```python
from build123d import *

# Parameters (mm, degrees)
BOSS_EXTRUDE1_DEPTH = 3.5814
BOSS_EXTRUDE2_DEPTH = 3.5814
SKETCH4_R           = 7.95
CUT_EXTRUDE2_DEPTH  = 4.5814
CUT_EXTRUDE4_REACH  = 5.581
CUT_EXTRUDE5_REACH  = 5.581


with BuildPart() as part:
    # Sketch1 → Boss-Extrude1 (new body)
    with BuildSketch(Plane(origin=(0, 0, 0), x_dir=(1, 0, 0), z_dir=(0, 1, 0))):
        Polygon((-25.0063, -13.0482), (25.0063, -13.0482), (25.0063, -2.05), (1.7907, -2.05), (1.7907, 2.05), (9.398, 2.05), (1.7907, 7.13), (-1.7907, 7.13), (-9.398, 2.05), (-1.7907, 2.05), (-1.7907, -2.05), (-25.0063, -2.05), align=None)
    extrude(amount=BOSS_EXTRUDE1_DEPTH)

    # Sketch3 → Boss-Extrude2 (add)
    with BuildSketch(Plane(origin=(0, 3.5814, 0), x_dir=(1, 0, 0), z_dir=(0, 1, 0))):
        Polygon((-25.0063, -2.05), (-25.0063, -13.0482), (25.0063, -13.0482), (25.0063, -2.05), (1.7907, -2.05), (1.7907, 2.05), (9.398, 2.05), (1.7907, 7.13), (-1.7907, 7.13), (-9.398, 2.05), (-1.7907, 2.05), (-1.7907, -2.05), align=None)
        with BuildLine():
            Line((25.0063, -13.0482), (-25.0063, -13.0482))
            ThreePointArc((-25.0063, -13.0482), (-16.136037163, -25.01193231), (-2.111127058, -20.000510342))
            ThreePointArc((-2.111127058, -20.000510342), (0, -18.87286389), (2.111127058, -20.000510342))
            ThreePointArc((2.111127058, -20.000510342), (16.136037163, -25.01193231), (25.0063, -13.0482))
        make_face()
    extrude(amount=-BOSS_EXTRUDE2_DEPTH)

    # Sketch4 → Cut-Extrude2 (cut, through all)
    with BuildSketch(Plane(origin=(0, 3.5814, 0), x_dir=(1, 0, 0), z_dir=(0, 1, 0))):
        with Locations((-13.5, -13.0482)):
            Circle(SKETCH4_R)
        with Locations((13.5, -13.0482)):
            Circle(SKETCH4_R)
    extrude(amount=-CUT_EXTRUDE2_DEPTH, mode=Mode.SUBTRACT)

    # Sketch5 → Cut-Extrude4 (cut, up to next)
    with BuildSketch(Plane(origin=(0, 3.5814, 0), x_dir=(1, 0, 0), z_dir=(0, 1, 0)), mode=Mode.PRIVATE) as cut_extrude4_sk1:
        with BuildLine():
            Line((-3.25, -3.8), (3.25, -3.8))
            ThreePointArc((3.25, -3.8), (4.487436867, -4.312563133), (5, -5.55))
            Line((5, -5.55), (10.858126279, -5.55))
            ThreePointArc((10.858126279, -5.55), (7.011340813, -8.454747926), (5.55, -13.0482))
            Line((5.55, -13.0482), (-5.55, -13.0482))
            ThreePointArc((-5.55, -13.0482), (-7.011340813, -8.454747926), (-10.858126279, -5.55))
            Line((-10.858126279, -5.55), (-5, -5.55))
            ThreePointArc((-5, -5.55), (-4.487436867, -4.312563133), (-3.25, -3.8))
        make_face()
    cut_extrude4_tool1 = extrude(cut_extrude4_sk1.sketch, amount=-CUT_EXTRUDE4_REACH, mode=Mode.PRIVATE) & part.part
    add(cut_extrude4_tool1.solids().sort_by_distance((0, 3.5814, 8.325803))[0], mode=Mode.SUBTRACT)

    # Sketch6 → Cut-Extrude5 (cut, up to next)
    with BuildSketch(Plane(origin=(0, 3.5814, 0), x_dir=(1, 0, 0), z_dir=(0, 1, 0)), mode=Mode.PRIVATE) as cut_extrude5_sk1:
        with BuildLine():
            Line((-18.450280122, -2.05), (-25.0063, -2.05))
            Line((-25.0063, -2.05), (-25.0063, -13.0482))
            ThreePointArc((-25.0063, -13.0482), (-23.242950275, -6.64621203), (-18.450280122, -2.05))
        make_face()
    cut_extrude5_tool1 = extrude(cut_extrude5_sk1.sketch, amount=-CUT_EXTRUDE5_REACH, mode=Mode.PRIVATE) & part.part
    add(cut_extrude5_tool1.solids().sort_by_distance((-23.17616, 3.5814, 4.635288))[0], mode=Mode.SUBTRACT)
    # Sketch6 → Cut-Extrude5 (cut, up to next)
    with BuildSketch(Plane(origin=(0, 3.5814, 0), x_dir=(1, 0, 0), z_dir=(0, 1, 0)), mode=Mode.PRIVATE) as cut_extrude5_sk2:
        with BuildLine():
            Line((25.0063, -13.0482), (25.0063, -2.05))
            Line((25.0063, -2.05), (18.450280122, -2.05))
            ThreePointArc((18.450280122, -2.05), (23.242950275, -6.64621203), (25.0063, -13.0482))
        make_face()
    cut_extrude5_tool2 = extrude(cut_extrude5_sk2.sketch, amount=-CUT_EXTRUDE5_REACH, mode=Mode.PRIVATE) & part.part
    add(cut_extrude5_tool2.solids().sort_by_distance((23.17616, 3.5814, 4.635288))[0], mode=Mode.SUBTRACT)


solid = part.part
```
Check sheet for the modelled part. Datum: model origin and axes. Units: mm. A direction names the side the tool comes from. Round coordinates to 2 decimals unless told otherwise and drop trailing zeros. Write each loop counter-clockwise with the first axis right and the second up, starting at its lowest first coordinate (ties: lowest second). Pieces come first, ordered by that corner, then holes. Notation, with made-up numbers: M 17,-24.5 L 71,-24.5 A23 ccw 71,-0.5 Z; hole C 70.5,-33 d5. An arc over 180 degrees is marked long. Write item = value, one per line. Start each with the question number.
1. Release check for a two-part mould opening along X. For faces 6 (the flat face through (-2, 3.581, 14)), 7 (the flat face through (5.648, 1.766, -4.554)), 8 (the cylindrical face through (19.8, 1.8, 17.9)) record: pulls with the +X half, pulls with the -X half, needs draft (parallel to the pull), parting line crosses it, or undercut.
2. Tool access check on faces 1 (the flat face through (6, 2, -2.05)), 2 (the flat face through (-2, 0, 14)), 3 (the flat face through (0, 2, -7.13)), 4 (the flat face through (8, 2, 5.55)), 5 (the flat face through (-6, 2, -2.05)). Record the directions out of +Z, -Z, +X, -X, +Y, -Y that give a thin tool (end or side, any length) a straight path to the whole face; none if there is none.
3. Section check D-D, the plane z = 16. Record the cut outline in (x, y).
4. Section check A-A, the plane y = 1.3. Record the cut outline in (x, z), then the cut area to 3 significant figures.
5. Gauge pin test, flat ends, axial feed: pin 1 (2 mm diameter, centred on x = 13, y = 2.5, fed in from -Z); pin 2 (9.5 mm diameter, centred on x = -13.5, z = 13.05, fed in from +Y); pin 3 (1.8 mm diameter, centred on x = 0, y = 1, fed in from +Z); pin 4 (1.1 mm diameter, centred on x = -4.5, y = 1, fed in from +Z). Record the tip position at first contact, or that the pin passes through.
6. Scan lines: line 1 (X direction, y = 0.7, z = 13); line 2 (Z direction, x = -7.5, y = 3.05); line 3 (X direction, y = 1.05, z = 19.5). Record each from-to range of solid material in increasing order. Write a range as [from, to].
7. Section check B-B, the plane x = 17.5. Record the cut outline in (y, z).
8. Section check C-C, the plane z = 11. Record the cut outline in (x, y).
Results found:
q1.face_6 = needs draft
q1.face_7 = pulls with the +X half
q1.face_8 = undercut
q2.face_1 = +X, +Y, -Y
q2.face_2 = +Z, -Z, +X, -X, -Y
q2.face_3 = -Z, +X, -X, +Y, -Y
q2.face_4 = +Y, -Y
q2.face_5 = -X, +Y, -Y
q3.outline = M -24.65,0 L -20.88,0 L -20.88,3.58 L -24.65,3.58 Z; M -6.12,0 L 6.12,0 L 6.12,3.58 L -6.12,3.58 Z; M 20.88,0 L 24.65,0 L 24.65,3.58 L 20.88,3.58 Z
q4.outline = M -18.45,2.05 L -1.79,2.05 L -1.79,-2.05 L -9.4,-2.05 L -1.79,-7.13 L 1.79,-7.13 L 9.4,-2.05 L 1.79,-2.05 L 1.79,2.05 L 18.45,2.05 A12.5 ccw long 2.11,20 A2.54 cw -2.11,20 A12.5 ccw long Z; hole M -10.86,5.55 L -5,5.55 A1.75 ccw -3.25,3.8 L 3.25,3.8 A1.75 ccw 5,5.55 L 10.86,5.55 A7.95 ccw long 5.55,13.05 L -5.55,13.05 A7.95 ccw long Z
q4.area = 559 mm^2
q5.pin_1 = 2.05
q5.pin_2 = through
q5.pin_3 = 19.04
q5.pin_4 = 23.09
q6.line_1 = [-25.01, -21.45], [21.45, 25.01]
q6.line_2 = [-3.32, -2.05], [2.05, 5.55], [18.26, 24.51]
q6.line_3 = [-23.21, -18.15], [-8.85, -1.67], [1.67, 8.85], [18.15, 23.21]
q7.outline = M 0,2.05 L 3.58,2.05 L 3.58,6.18 L 0,6.18 Z; M 0,19.92 L 3.58,19.92 L 3.58,24.51 L 0,24.51 Z
q8.outline = M -24.84,0 L -21.18,0 L -21.18,3.58 L -24.84,3.58 Z; M 21.18,0 L 24.84,0 L 24.84,3.58 L 21.18,3.58 Z
